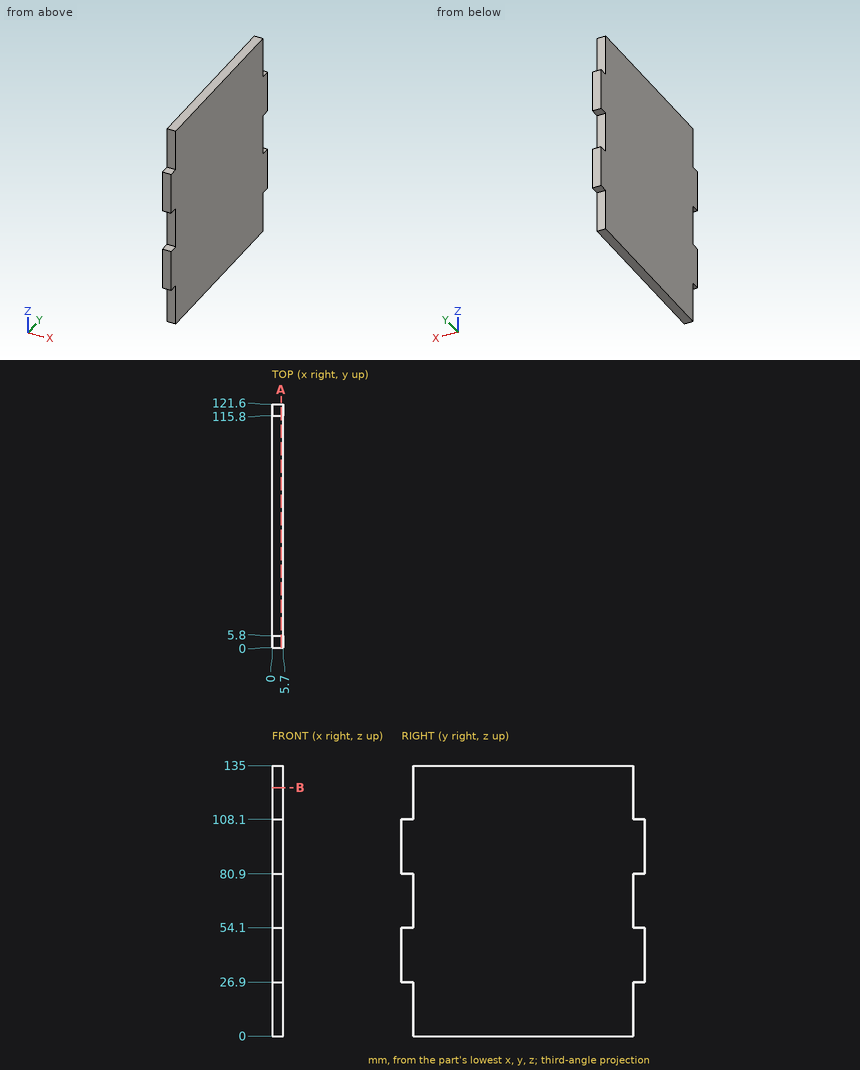
Geometry: see drawing. Coordinates: mm, zero at the bounding-box minimum. Coordinates: 2 decimals unless noted, no trailing zeros. Loops run counter-clockwise (first coordinate to the right, second up) from the corner with the lowest first, then second, coordinate; pieces in that order, holes last. Notation, with made-up numbers: (-32, -12) - (-3, -12) arc R27 cw to (-3, 19) - close; hole circle Ø3 at (-33.5, 40). An arc over 180 degrees is marked (long way). Put each result on its own line as item: value. Start each with the question number.
Q1. Cut plane B-B, the plane z = 124. Return loops of the section in (x, y).
Q2. Cut plane A-A, the plane x = 4.5. Return loops of the section in (y, z).
Q3. Line query: line 1 (Y direction, x = 3.5, z = 18.5). Output: solid intervals per line, ascending.
Q4. Pin query (flat end, axial travel): pin 1 Ø3 at (x, y) = (4, 3) entering from +Z; pin 2 Ø1.7 at (x, y) = (2, 119) entering from -Z; pin 3 Ø1.7 at (x, z) = (3, 67.5) entering from -Y. Return the tip coordinate at first contact, or that it passes through.
Filled sheet:
1. outline: (0, 5.8) - (5.7, 5.8) - (5.7, 115.8) - (0, 115.8) - close
2. outline: (0, 26.9) - (5.8, 26.9) - (5.8, 0) - (115.8, 0) - (115.8, 26.9) - (121.6, 26.9) - (121.6, 54.1) - (115.8, 54.1) - (115.8, 80.9) - (121.6, 80.9) - (121.6, 108.1) - (115.8, 108.1) - (115.8, 135) - (5.8, 135) - (5.8, 108.1) - (0, 108.1) - (0, 80.9) - (5.8, 80.9) - (5.8, 54.1) - (0, 54.1) - close
3. line 1: 5.8 to 115.8
4. pin 1: z = 108.1
4. pin 2: z = 26.9
4. pin 3: y = 5.8
